```python
from build123d import *

# Parameters (mm, degrees)
SKETCH1_R           = 1.5
SKETCH1_R_2         = 2.25
SKETCH1_W           = 4
SKETCH1_H           = 2
BOSS_EXTRUDE1_DEPTH = 2
BOSS_EXTRUDE2_DEPTH = 2
SKETCH4_R           = 1.5
CUT_EXTRUDE1_DEPTH  = 2


with BuildPart() as part:
    # Sketch1 → Boss-Extrude1 (new body)
    with BuildSketch(Plane(origin=(0, 0, 0), x_dir=(1, 0, 0), z_dir=(0, 1, 0))):
        Polygon((0, 0), (5, 0), (5, -2), (9, -2), (9, 0), (12.5, 0), (12.5, 2), (11.4, 2), (11.4, 4.3), (12.5, 4.3), (12.5, 6), (15.5, 6), (15.5, 4.3), (16.6, 4.3), (16.6, 2), (15.5, 2), (15.5, 0), (19, 0), (19, -2), (23, -2), (23, 0), (28, 0), (28, 66), (0, 66), align=None)
        with Locations(Location((14, 64, 0), (0, 0, 270))):
            Circle(SKETCH1_R, mode=Mode.SUBTRACT)
        with Locations(Location((14, 23.49, 0), (0, 0, 270))):
            Circle(SKETCH1_R_2, mode=Mode.SUBTRACT)
        with Locations((7, 64)):
            Rectangle(SKETCH1_W, SKETCH1_H, mode=Mode.SUBTRACT)
        with Locations((21, 64)):
            Rectangle(SKETCH1_W, SKETCH1_H, mode=Mode.SUBTRACT)
    extrude(amount=BOSS_EXTRUDE1_DEPTH)

    # Sketch2 → Boss-Extrude2 (add)
    with BuildSketch(Plane(origin=(0, 2, 0), x_dir=(1, 0, 0), z_dir=(0, 1, 0))):
        with BuildLine():
            Line((0, 66), (28, 66))
            ThreePointArc((28, 66), (34.819271185, 129.864214399), (70.378490249, 183.349560802))
            ThreePointArc((70.378490249, 183.349560802), (70.223472253, 188.82876401), (64.776007814, 189.43772177))
            ThreePointArc((64.776007814, 189.43772177), (17.177564343, 135.700793296), (0, 66))
        make_face()
    extrude(amount=-BOSS_EXTRUDE2_DEPTH)

    # Sketch4 → Cut-Extrude1 (cut)
    with BuildSketch(Plane(origin=(0, 2, 0), x_dir=(1, 0, 0), z_dir=(0, 1, 0))):
        with Locations(Location((44.36627387, 163, 0), (0, 0, 270))):
            Circle(SKETCH4_R)
        with BuildLine():
            Line((49.278104547, 158.611243867), (90.336581865, 196.333434103))
            Line((90.336581865, 196.333434103), (75.550012159, 212.427781571))
            Line((75.550012159, 212.427781571), (35.469078733, 175.603702981))
            Line((35.469078733, 175.603702981), (39.454443193, 167.388756133))
            ThreePointArc((39.454443193, 167.388756133), (48.755030003, 167.911830677), (49.278104547, 158.611243867))
        make_face()
    extrude(amount=-CUT_EXTRUDE1_DEPTH, mode=Mode.SUBTRACT)


solid = part.part
```
Part model, mm, in its own coordinate system. Coordinates: 2 decimals unless noted, no trailing zeros. Write each loop counter-clockwise with the first axis right and the second up, starting at its lowest first coordinate (ties: lowest second). Pieces come first, ordered by that corner, then holes.
Item 1: Pin check, flat tips, straight feed: pin 1 (1 mm diameter, centred on y = 1, z = -41, fed in from +X); pin 2 (2.5 mm diameter, centred on x = 14, z = -64, fed in from -Y); pin 3 (0.9 mm diameter, centred on x = 12, y = 0.5, fed in from +Z); pin 4 (1 mm diameter, centred on x = 21, y = 1, fed in from -Z). Stop position of each tip, or through.
Item 2: Slice it at A-A (z = -23.49). Write the cut outline in (x, y), and give its area (3 significant figures).
Item 3: Slice it at B-B (x = 14). Write the cut outline in (y, z).
Item 4: Mould opens along X. For faces 1 (the face through (14.45, 0.99, -62.57)), 2 (the face through (44.82, 1.01, -161.57)), 3 (the face through (19, 2, -85)), 4 (the face through (10.53, 1.01, -121.21)) say: released by +X, released by -X, zero draft, split by the parting line, or undercut.
Item 5: Slice it at D-D (z = -46). Write the cut outline in (x, y), and give its area (3 significant figures).
Item 6: Slice it at C-C (y = 0.9). Count the separate pieces of the cut face and the enclosed holes in it, and give its area (3 significant figures).
Item 7: Probe line 1 (X direction, y = 0.55, z = -64); line 2 (X direction, y = 0.5, z = -23.49); line 3 (X direction, y = 1.1, z = -35.5). List the from-to ranges inside material, lowest first.
Results found:
1. pin 1: stops at x = 28
1. pin 2: passes through
1. pin 3: stops at z = 0
1. pin 4: stops at z = -143.38
2. outline: (0, 0) - (11.75, 0) - (11.75, 2) - (0, 2) - close; (16.25, 0) - (28, 0) - (28, 2) - (16.25, 2) - close
2. area: 47.0 mm2
3. outline: (0, -129.28) - (2, -129.28) - (2, -65.5) - (0, -65.5) - close; (0, -62.5) - (2, -62.5) - (2, -25.74) - (0, -25.74) - close; (0, -21.24) - (2, -21.24) - (2, -6) - (0, -6) - close
4. face 1: undercut
4. face 2: undercut
4. face 3: zero draft
4. face 4: released by -X
5. outline: (0, 0) - (28, 0) - (28, 2) - (0, 2) - close
5. area: 56.0 mm2
6. separate pieces: 1
6. enclosed holes: 5
6. area: 4,030 mm2
7. line 1: x = 0 to 5, 9 to 12.5, 15.5 to 19, 23 to 28
7. line 2: x = 0 to 11.75, 16.25 to 28
7. line 3: x = 0 to 28
